Verification items for the finished model (mm, model axes). Face numbers are marked on the shaded views. A direction names the side the tool comes from. Coordinates: 2 decimals unless noted, no trailing zeros. Order: outer loops, then holes, each group sorted by start corner. A loop starts at its lowest first (then second) coordinate and runs counter-clockwise, first axis right, second up.
Q1. Cross-section at B-B, the plane x = 2.75. Record the boundary of the cut face in (y, z) (3 decimals), and give its area (3 significant figures).
Q2. Cross-section at A-A, the plane y = 0.8. Record the boundary of the cut face in (x, z) (3 decimals).
Q3. Set-up check for the marked faces 4 and 5: record each of +Z, -Z, +X, -X, +Y, -Y from which the full face is reachable in a straight line by a thin tool's end or side.
Q4. Thickness scan on line 1 (X direction, y = 1.05, z = -2.5) (3 decimals); line 2 (Z direction, x = 10.5, y = 1.15) (3 decimals); line 3 (Z direction, x = 4.25, y = 1.1) (3 decimals). Record the ranges inside material, lowest first.
Q5. Cross-section at C-C, the plane z = -6.35. Record the boundary of the cut face in (x, y) (3 decimals).
Q6. Draft check along Z on the marked faces 1, 2 and 3. Enter one of: pulls with the +Z half, pulls with the -Z half, needs draft (parallel to the pull), parting line crosses it, or undercut.
Q7. Depth check by flat-ended pin: P1, Ø1.5, axis at x = 10, z = -3, coming from the +Y side. Enter the tip coordinate at first touch or a pass-through.
Q8. Cross-section at D-D, the plane z = -1.75. Record the boundary of the cut face in (x, y) (3 decimals).
from build123d import *

# Parameters (mm, degrees)
SKETCH1_W           = 12.7
SKETCH1_H           = 12.7
BOSS_EXTRUDE1_DEPTH = 2.54
FILLET1_R           = 0.635
SHELL1_START        = 0.635
SHELL1_OUTLINE_W    = 1.905
SHELL1_OUTLINE_H    = 11.43
SHELL1_DEPTH        = 11.43
SKETCH2_R           = 2.54
BOSS_EXTRUDE2_DEPTH = 1.905
SKETCH4_W           = 0.325641025
SKETCH4_H           = 4.111217948
BOSS_EXTRUDE4_DEPTH = 0.00254


# Read off the part's stored shape, not the designer's step: Shell1
with BuildPart() as part:
    # Sketch1 → Boss-Extrude1 (new body)
    with BuildSketch(Plane(origin=(0, 0, 0), x_dir=(1, 0, 0), z_dir=(0, 1, 0))):
        with Locations((6.35, 6.35)):
            Rectangle(SKETCH1_W, SKETCH1_H)
    extrude(amount=BOSS_EXTRUDE1_DEPTH)

    # Fillet1
    fillet1_edges = [part.edges().sort_by_distance(p)[0] for p in [
        (0, 1.27, -12.7),
        (12.7, 1.27, -12.7),
        (12.7, 1.27, 0),
        (0, 1.27, 0),
    ]]
    fillet(fillet1_edges, radius=FILLET1_R)

    # Shell1 outline → Shell1 (cut)
    with BuildSketch(Plane.YZ.offset(SHELL1_START)):
        with Locations((0.9525, -6.35)):
            Rectangle(SHELL1_OUTLINE_W, SHELL1_OUTLINE_H)
    extrude(amount=SHELL1_DEPTH, mode=Mode.SUBTRACT)

    # Sketch2 → Boss-Extrude2 (add)
    with BuildSketch(Plane(origin=(0, 1.905, 0), x_dir=(-1, 0, 0), z_dir=(0, -1, 0))):
        with Locations(Location((-6.35, 6.35, 0), (0, 0, 270))):
            Circle(SKETCH2_R)
    extrude(amount=BOSS_EXTRUDE2_DEPTH)

    # Sketch4 → Boss-Extrude4 (add)
    with BuildSketch(Plane(origin=(0, 2.54, 0), x_dir=(1, 0, 0), z_dir=(0, 1, 0))):
        Polygon((7.464964343, 1.970128205), (7.033744391, 1.970128205), (5.628145433, 5.796410256), (6.059365385, 5.796410256), align=None)
        with Locations((6.382564102, 9.074801282)):
            Rectangle(SKETCH4_W, SKETCH4_H)
    extrude(amount=BOSS_EXTRUDE4_DEPTH)


solid = part.part
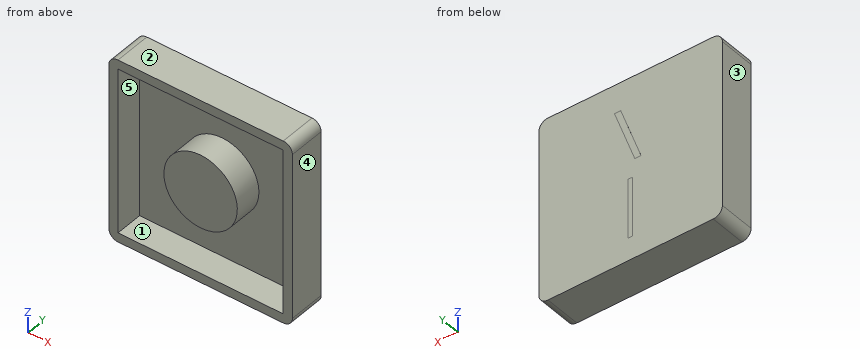
Check values:
1. outline: (0, -12.7) - (2.54, -12.7) - (2.54, 0) - (0, 0) - (0, -0.635) - (1.905, -0.635) - (1.905, -12.065) - (0, -12.065) - close
1. area: 10.5 mm2
2. outline: (0, -12.065) arc R0.635 ccw to (0.635, -12.7) - (12.065, -12.7) arc R0.635 ccw to (12.7, -12.065) - (12.7, -0.635) arc R0.635 ccw to (12.065, 0) - (0.635, 0) arc R0.635 ccw to (0, -0.635) - close; circle Ø5.08 at (6.35, -6.35); hole (0.635, -12.065) - (12.065, -12.065) - (12.065, -0.635) - (0.635, -0.635) - close
3. face 4: +Z, -Z, +X, +Y, -Y
3. face 5: -Y
4. line 1: x = 0 to 0.635, 12.065 to 12.7
4. line 2: z = -12.7 to -12.065, -0.635 to 0
4. line 3: z = -12.7 to -12.065, -7.779 to -4.921, -0.635 to 0
5. outline: (0, 0) - (0.635, 0) - (0.635, 1.905) - (3.81, 1.905) - (3.81, 0) - (8.89, 0) - (8.89, 1.905) - (12.065, 1.905) - (12.065, 0) - (12.7, 0) - (12.7, 2.54) - (0, 2.54) - close
6. face 1: undercut
6. face 2: pulls with the +Z half
6. face 3: needs draft
7. P1: stops at y = 2.54
8. outline: (0, 0) - (0.635, 0) - (0.635, 1.905) - (12.065, 1.905) - (12.065, 0) - (12.7, 0) - (12.7, 2.54) - (0, 2.54) - close
